Input: part model. Units: mm. Frame: model coordinates. Face numbers are marked on the shaded views. Coordinates: 2 decimals unless noted, no trailing zeros. Write each loop counter-clockwise with the first axis right and the second up, starting at its lowest first coordinate (ties: lowest second). Pieces come first, ordered by that corner, then holes.
1) Pin query (flat end, axial travel): pin 1 Ø5 at (y, z) = (7, -6) entering from +X; pin 2 Ø2 at (y, z) = (5.5, 0.5) entering from +X; pin 3 Ø8 at (x, z) = (-7, -3) entering from +Y. Return the tip coordinate at first contact, or that it passes through.
2) Section query B-B (y = 0). Output: boundary loops of the cut face in (x, z), then the cut area to 3 significant figures.
3) Section query C-C (z = 4). Output: boundary loops of the cut face in (x, y).
4) Line query: L1, parallel to Y at x = 0, z = -2.75; L2, parallel to X at y = 7, z = -5; L3, parallel to Z at x = 0, y = 9.25. Output: solid intervals per line, ascending.
5) Section query D-D (z = -2). Output: boundary loops of the cut face in (x, y), then the cut area to 3 significant figures.
6) Section query A-A (x = 0). Output: boundary loops of the cut face in (y, z), then the cut area to 3 significant figures.
7) Draft query along X for the marked faces 1, 2 and 3. Return one class per face: pulls with the +X half, pulls with the -X half, needs draft (parallel to the pull), parting line crosses it, or undercut.
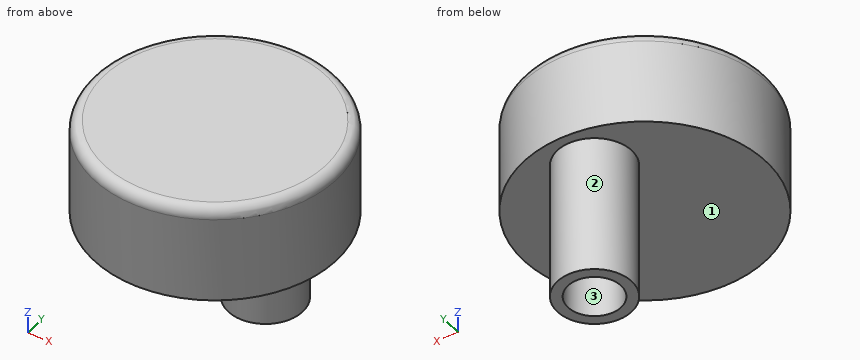
from build123d import *

# Parameters (mm, degrees)
F0_R     = 11.4
F1_DEPTH = 9
F2_R     = 3.5
F2_R_2   = 2.5
F3_DEPTH = 13
F4_R     = 1


with BuildPart() as f1:
    # F0 (on Top) → F1 (new body)
    with BuildSketch(Plane.XY):
        Circle(F0_R)
    extrude(amount=F1_DEPTH)

    # F2 (on face) → F3 (join)
    with BuildSketch(Plane(origin=(0, 0, 0), x_dir=(1, 0, 0), z_dir=(0, 0, -1))):
        with Locations((0, -7)):
            Circle(F2_R)
        with Locations((0, -7)):
            Circle(F2_R_2, mode=Mode.SUBTRACT)
    extrude(amount=F3_DEPTH)

    # F4
    f4_edges = [f1.edges().sort_by_distance(p)[0] for p in [
        (-11.4, 0, 9),
    ]]
    fillet(f4_edges, radius=F4_R)


solid = f1.part
Answer:
1. pin 1: stops at x = 3.5
1. pin 2: stops at x = 10.47
1. pin 3: stops at y = 10.54
2. outline: (-11.4, 0) - (11.4, 0) - (11.4, 8) arc R1 ccw to (10.4, 9) - (-10.4, 9) arc R1 ccw to (-11.4, 8) - close
2. area: 205 mm2
3. outline: circle Ø22.8 at (0, 0)
4. L1: y = 3.5 to 4.5, 9.5 to 10.5
4. L2: x = -3.5 to -2.5, 2.5 to 3.5
4. L3: z = 0 to 9
5. outline: circle Ø7 at (0, 7); hole circle Ø5 at (0, 7)
5. area: 18.8 mm2
6. outline: (-11.4, 0) - (3.5, 0) - (3.5, -13) - (4.5, -13) - (4.5, 0) - (9.5, 0) - (9.5, -13) - (10.5, -13) - (10.5, 0) - (11.4, 0) - (11.4, 8) arc R1 ccw to (10.4, 9) - (-10.4, 9) arc R1 ccw to (-11.4, 8) - close
6. area: 231 mm2
7. face 1: needs draft
7. face 2: parting line crosses it
7. face 3: undercut
